from build123d import *

# Parameters (mm, degrees)
F0_R     = 215.9
F1_DEPTH = 50.8
F2_R     = 120.65
F2_R_2   = 85.09
F3_DEPTH = 20.32
F4_R     = 12.7
F5_DEPTH = 50.801


with BuildPart() as f1:
    # F0 (on Top) → F1 (new body)
    with BuildSketch(Plane.XY):
        Circle(F0_R)
    extrude(amount=F1_DEPTH)

    # F2 (on face) → F3 (cut)
    with BuildSketch(Plane.XY.offset(50.8)):
        Circle(F2_R)
        Circle(F2_R_2, mode=Mode.SUBTRACT)
    extrude(amount=-F3_DEPTH, mode=Mode.SUBTRACT)

    # F4 (on face) → F5 (cut, through all)
    with BuildSketch(Plane.XY.offset(50.8)):
        Circle(F4_R)
    extrude(amount=-F5_DEPTH, mode=Mode.SUBTRACT)


solid = f1.part
Geometry: final body of the model. Coordinates: model frame, mm. A direction names the side the tool comes from. Give positions to 0.01 mm unless a question says otherwise; leave off trailing zeros. Write each loop counter-clockwise with the first axis right and the second up, starting at its lowest first coordinate (ties: lowest second). Pieces come first, ordered by that corner, then holes.
(1) Cut plane A-A, the plane y = 0. Return loops of the section in (x, z), then the cut area to 3 significant figures.
(2) Access query for faces 4 (the cylindrical face through (-67.52, -51.78, 40.78)), 5 (the cylindrical face through (-2.75, -12.4, 25.76)). Directions: +Z, -Z, +X, -X, +Y, -Y. A direction counts if a zero-diameter tool reaches every point of the face in a straight line with its end or side. Return the directions, or none.
(3) Cut plane D-D, the plane z = 18. Return loops of the section in (x, y).
(4) First-contact query: P1, Ø3, axis at y = -153.5, z = 36.5, coming from the +X side; P2, Ø1, axis at y = 84, z = 37.5, coming from the +X side; P3, Ø2, axis at x = 35, z = 25, coming from the -Y side; P4, Ø3, axis at x = 37.5, y = -13, coming from the -Z side. Flat tips, straight axial feed; report the tip coordinate or a pass-through.
(5) Ray query, line 1 (Y direction, x = 0, z = 36); line 2 (Y direction, x = 70, z = 43.5); line 3 (Y direction, x = 0, z = 10). Return the intervals inside material, ascending.
(6) Mould query, pull axis Y, two halves, no side actions, for faces 1 (the flat face through (-1, -18, 50.8)), 2 (the cylindrical face through (-120.533, 5.305, 40.782)), 3 (the cylindrical face through (-159.127, 145.915, 25.044)). Classes: released by +Y, released by -Y, zero draft, split by the parting line, or undercut.
(7) Cut plane C-C, the plane x = 59. Return loops of the section in (y, z).
Values follow:
1. outline: (-215.9, 0) - (-12.7, 0) - (-12.7, 50.8) - (-85.09, 50.8) - (-85.09, 30.48) - (-120.65, 30.48) - (-120.65, 50.8) - (-215.9, 50.8) - close; (12.7, 0) - (215.9, 0) - (215.9, 50.8) - (120.65, 50.8) - (120.65, 30.48) - (85.09, 30.48) - (85.09, 50.8) - (12.7, 50.8) - close
1. area: 19,200 mm2
2. face 4: +Z
2. face 5: +Z, -Z
3. outline: circle Ø431.8 at (0, 0); hole circle Ø25.4 at (0, 0)
4. P1: stops at x = 153.33
4. P2: stops at x = 199.1
4. P3: stops at y = -213.21
4. P4: stops at z = 0
5. line 1: y = -215.9 to -120.65, -85.09 to -12.7, 12.7 to 85.09, 120.65 to 215.9
5. line 2: y = -204.24 to -98.27, -48.38 to 48.38, 98.27 to 204.24
5. line 3: y = -215.9 to -12.7, 12.7 to 215.9
6. face 1: zero draft
6. face 2: undercut
6. face 3: split by the parting line
7. outline: (-207.68, 0) - (207.68, 0) - (207.68, 50.8) - (105.24, 50.8) - (105.24, 30.48) - (61.31, 30.48) - (61.31, 50.8) - (-61.31, 50.8) - (-61.31, 30.48) - (-105.24, 30.48) - (-105.24, 50.8) - (-207.68, 50.8) - close
